Design review of the part shown in the three views and the two pictorial views. Dimensions are in mm from the part's minimum x, y and z. Give positions to 0.01 mm unless a question says otherwise; leave off trailing zeros. Write each loop counter-clockwise with the first axis right and the second up, starting at its lowest first coordinate (ties: lowest second). Pieces come first, ordered by that corner, then holes.
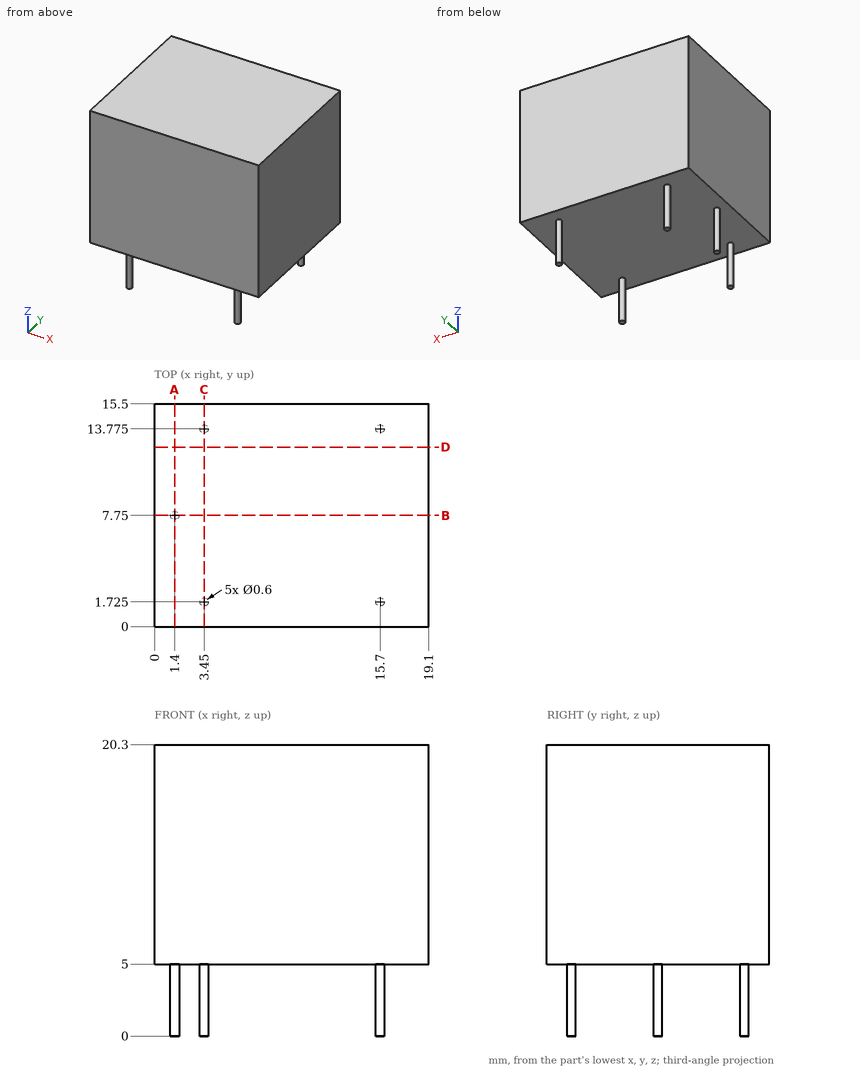
(1) Consider section B-B, the plane y = 7.75. Give the boundary of the cut face in (x, z).
Resolved:
outline: (0, 5) - (1.1, 5) - (1.1, 0) - (1.7, 0) - (1.7, 5) - (19.1, 5) - (19.1, 20.3) - (0, 20.3) - close
(2) Consider section D-D, the plane y = 12.5. Give the boundary of the cut face in (x, z), then the cut area to 3 significant figures.
Resolved:
outline: (0, 5) - (19.1, 5) - (19.1, 20.3) - (0, 20.3) - close
area: 292 mm2
(3) Consider section C-C, the plane x = 3.45. Give the boundary of the cut face in (y, z) (3 decimals), then the cut area to 3 significant figures.
Resolved:
outline: (0, 5) - (1.425, 5) - (1.425, 0) - (2.025, 0) - (2.025, 5) - (13.475, 5) - (13.475, 0) - (14.075, 0) - (14.075, 5) - (15.5, 5) - (15.5, 20.3) - (0, 20.3) - close
area: 243 mm2
(4) Clearance check with flat-ended pins moving along their axes: P1, Ø4, axis at x = 2, z = 2.5, coming from the +Y side (3 decimals); P2, Ø4.5, axis at x = 11, y = 5.5, coming from the -Z side. State where each tip first meets the part, or that it passes through.
Resolved:
P1: stops at y = 14.075
P2: stops at z = 5
(5) To check wall thickness, follow L1, parallel to Z at x = 17.75, y = 3.25. State the ranges of the line that lie inside material, in increasing order.
Resolved:
L1: z = 5 to 20.3
(6) Consider section A-A, the plane x = 1.4. Give the boundary of the cut face in (y, z).
Resolved:
outline: (0, 5) - (7.45, 5) - (7.45, 0) - (8.05, 0) - (8.05, 5) - (15.5, 5) - (15.5, 20.3) - (0, 20.3) - close
